```python
from build123d import *

# Parameters (mm, degrees)
SKETCH1_W               = 9.525
SKETCH1_H               = 9.525
BOSS_EXTRUDE1_DEPTH     = 42.8625
F_1_4_CLEARANCE_HOLE1_D = 6.7564
F_4_CLEARANCE_HOLE1_D   = 3.2639


with BuildPart() as part:
    # Sketch1 → Boss-Extrude1 (new, symmetric)
    with BuildSketch(Plane.XY):
        Rectangle(SKETCH1_W, SKETCH1_H)
    extrude(amount=BOSS_EXTRUDE1_DEPTH, both=True)

    # 1/4 Clearance Hole1 (through all)
    with Locations(Plane(origin=(0, 4.7625, 0), x_dir=(1, 0, 0), z_dir=(0, 1, 0))):
        with Locations((0, 37.1729)):
            f_1_4_clearance_hole1 = Hole(F_1_4_CLEARANCE_HOLE1_D / 2)

    # Mirror1: 1/4 Clearance Hole1 across plane
    add(f_1_4_clearance_hole1.mirror(Plane.XY), mode=Mode.SUBTRACT)

    # #4 Clearance Hole1 (through all)
    with Locations(Plane(origin=(4.7625, 0, 0), x_dir=(0, 0, -1), z_dir=(1, 0, 0))):
        with Locations((9.525, 0), (25.4, 0)):
            f_4_clearance_hole1 = Hole(F_4_CLEARANCE_HOLE1_D / 2)

    # Mirror2: #4 Clearance Hole1 across plane
    add(f_4_clearance_hole1.mirror(Plane.XY), mode=Mode.SUBTRACT)


solid = part.part
```
Can you work these out from the model? Positions are in its coordinate system, mm. Coordinates: 2 decimals unless noted, no trailing zeros. Write each loop counter-clockwise with the first axis right and the second up, starting at its lowest first coordinate (ties: lowest second). Pieces come first, ordered by that corner, then holes. Notation, with made-up numbers: M 44.25,85 L 59.25,85 A15 ccw 59.25,99 Z; hole C 8.25,44 d9. An arc over 180 degrees is marked long. Write item = value, one per line. Start each with the question number.
Q1. If we section it at D-D, the plane y = 4: Write out the boundary of the cut face in (x, z), then the cut area to 3 significant figures.
Q2. Thinking about a two-plate mould opening in Z: for faces 1 (the face through (4.762, 0, 1)), 2 (the face through (0, 0, 42.862)), 3 (the face through (-0.067, 0.072, 11.155)), which applies, released by +Z, released by -Z, zero draft, split by the parting line, or undercut?
Q3. If I drill on L1, parallel to Y at x = -2.25, z = 25.4; L2, parallel to Z at x = 1.75, y = 3.5; L3, parallel to Z at x = 2.25, y = 3.5, over which ranges is the centre line in solid material (lowest first)? Write a range as [from, to].
Q4. If we section it at A-A, the plane x = 0: Write out the boundary of the cut face in (y, z) (1 decimal), then the cut area to 3 significant figures.
Q5. If we section it at C-C, the plane y = 0.75: Write out the boundary of the cut face in (x, z), then the cut area to 3 significant figures.
Q6. If we section it at B-B, the plane z = -25.4: Write out the boundary of the cut face in (x, y), then the cut area to 3 significant figures.
Q7. I'm going to push a flat-ended pin straight in: pin 1 (2 mm diameter, centred on y = 0, z = 9.525, fed in from -X). Where does the tip first touch, or does it pass through?
Check sheet entries:
q1.outline = M -4.76,-42.86 L 4.76,-42.86 L 4.76,42.86 L -4.76,42.86 Z; hole C 0,-37.17 d6.76; hole C 0,37.17 d6.76
q1.area = 745 mm²
q2.face_1 = zero draft
q2.face_2 = released by +Z
q2.face_3 = undercut
q3.L1 = [-4.76, -1.63], [1.63, 4.76]
q3.L2 = [-42.86, -40.06], [-34.28, 34.28], [40.06, 42.86]
q3.L3 = [-42.86, -39.69], [-34.65, 34.65], [39.69, 42.86]
q4.outline = M -4.8,-42.9 L 4.8,-42.9 L 4.8,-40.6 L -4.8,-40.6 Z; M -4.8,-33.8 L 4.8,-33.8 L 4.8,33.8 L -4.8,33.8 Z; M -4.8,40.6 L 4.8,40.6 L 4.8,42.9 L -4.8,42.9 Z; hole C 0,-25.4 d3.3; hole C 0,-9.5 d3.3; hole C 0,9.5 d3.3; hole C 0,25.4 d3.3
q4.area = 654 mm²
q5.outline = M -4.76,-42.86 L 4.76,-42.86 L 4.76,-26.85 L -4.76,-26.85 Z; M -4.76,-23.95 L 4.76,-23.95 L 4.76,-10.97 L -4.76,-10.97 Z; M -4.76,-8.08 L 4.76,-8.08 L 4.76,8.08 L -4.76,8.08 Z; M -4.76,10.97 L 4.76,10.97 L 4.76,23.95 L -4.76,23.95 Z; M -4.76,26.85 L 4.76,26.85 L 4.76,42.86 L -4.76,42.86 Z; hole C 0,-37.17 d6.76; hole C 0,37.17 d6.76
q5.area = 634 mm²
q6.outline = M -4.76,-4.76 L 4.76,-4.76 L 4.76,-1.63 L -4.76,-1.63 Z; M -4.76,1.63 L 4.76,1.63 L 4.76,4.76 L -4.76,4.76 Z
q6.area = 59.6 mm²
q7.pin_1 = through
